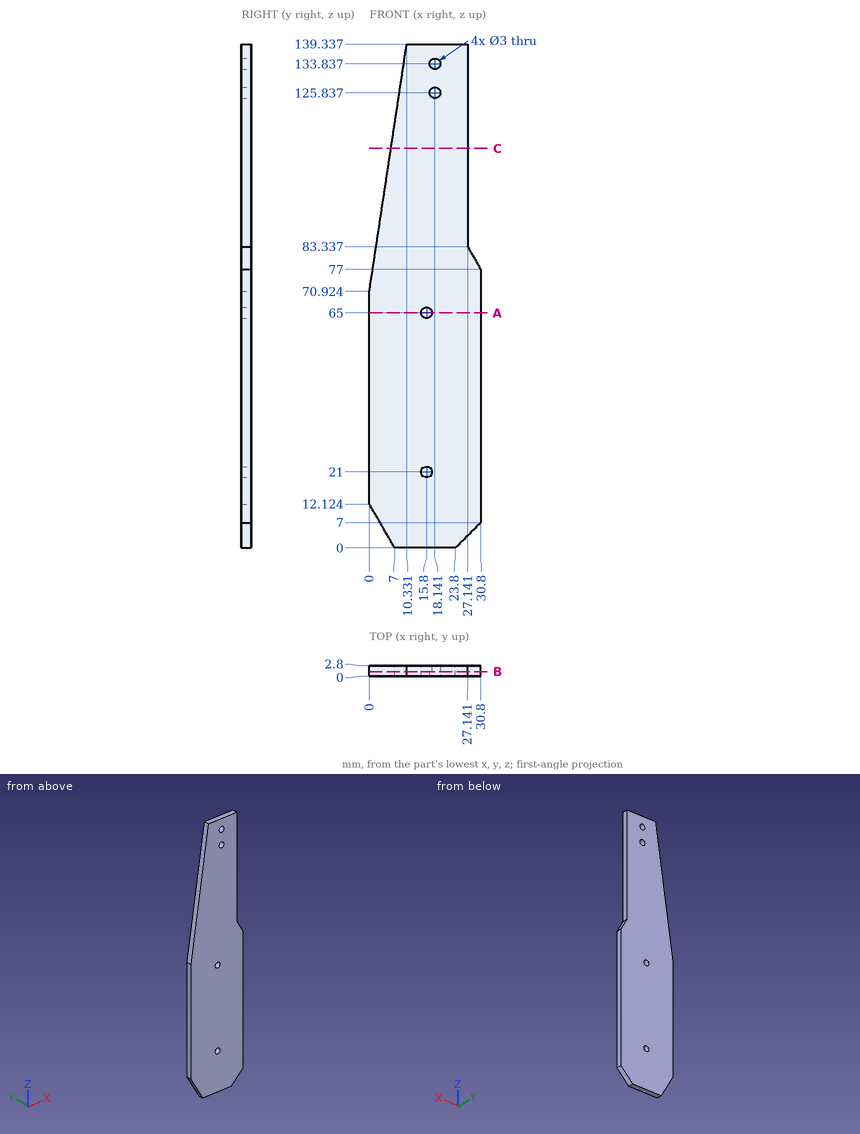
Print and shaded views of the part. All mm, measured from the part's lowest x, y and z. Give positions to 0.01 mm unless a question says otherwise; leave off trailing zeros. Write each loop counter-clockwise with the first axis right and the second up, starting at its lowest first coordinate (ties: lowest second). Pieces come first, ordered by that corner, then holes. Notation, with made-up numbers: (-16.75, 20) - (-6.75, 20) arc R34 ccw to (-6.75, 51) - close; hole circle Ø11 at (-30, 77). An arc over 180 degrees is marked (long way). One line per question, with ' | ' between items. Start each with the question number.
(1) Wall check: line 1 along Z through (x, y) = (16, 2.65); line 2 along X through (y, z) = (1.15, 21); line 3 along Z through (x, y) = (24, 0.15). Give the ranges that are in metal, low to high. Write a range as from..to.
(2) Slice it at A-A on z = 65. Write the cut outline in (x, y).
(3) Slice it at B-B on y = 1.2. Write the cut outline in (x, z) (1 decimal).
(4) Slice it at C-C on z = 110.5. Write the cut outline in (x, y).
Results below:
1) line 1: 0..19.51, 22.49..63.51, 66.49..139.34 | line 2: 0..14.3, 17.3..30.8 | line 3: 0.2..139.34
2) outline: (0, 0) - (14.3, 0) - (14.3, 2.8) - (0, 2.8) - close; (17.3, 0) - (30.8, 0) - (30.8, 2.8) - (17.3, 2.8) - close
3) outline: (0, 12.1) - (7, 0) - (23.8, 0) - (30.8, 7) - (30.8, 77) - (27.1, 83.3) - (27.1, 139.3) - (10.3, 139.3) - (0, 70.9) - close; hole circle Ø3 at (15.8, 21); hole circle Ø3 at (15.8, 65); hole circle Ø3 at (18.1, 125.8); hole circle Ø3 at (18.1, 133.8)
4) outline: (5.98, 0) - (27.14, 0) - (27.14, 2.8) - (5.98, 2.8) - close
